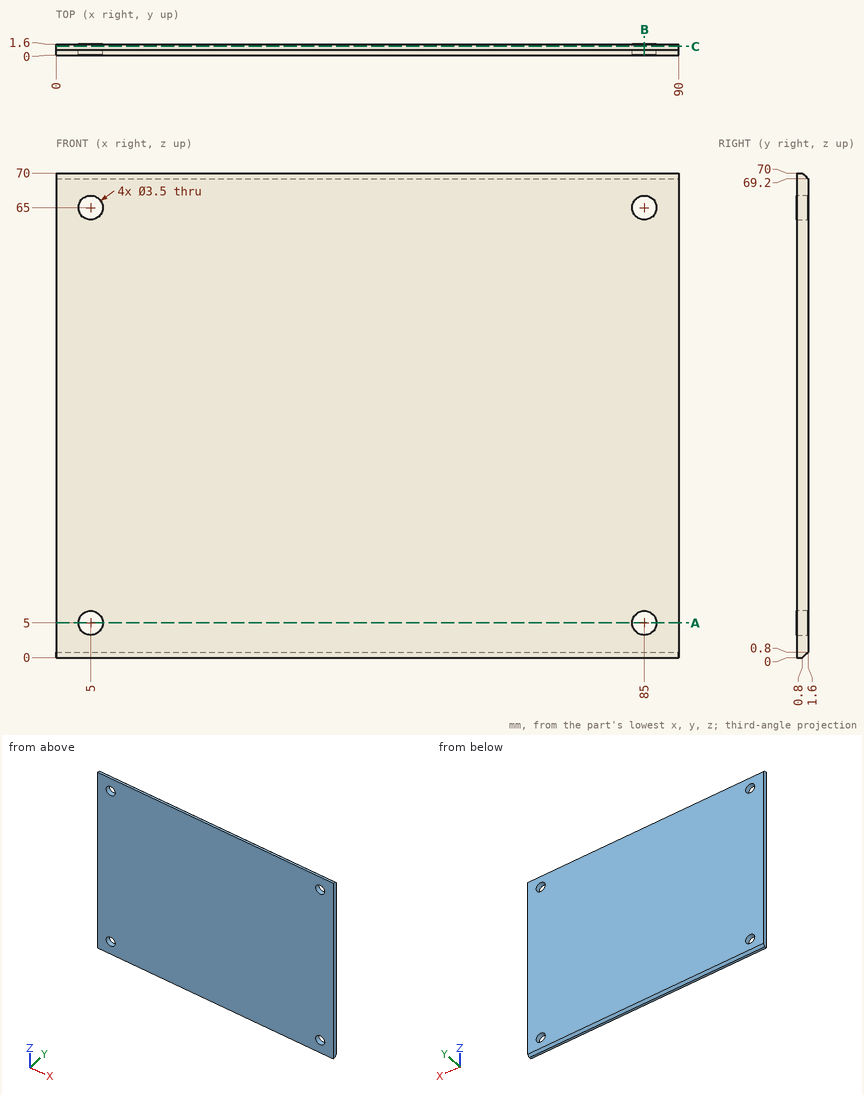
For this review, use the dimensioned drawing (mm, ordinates from the lowest corner) and the shaded views. Round coordinates to 2 decimals unless told otherwise and drop trailing zeros. Write each loop counter-clockwise with the first axis right and the second up, starting at its lowest first coordinate (ties: lowest second). Pieces come first, ordered by that corner, then holes. Notation, with made-up numbers: M -19,53 L -8,53 A19 ccw -8,79 Z; hole C 29,43 d8. An arc over 180 degrees is marked long. Use CSV: the item, a comma, the result in double quotes. Start each with the question number.
(1) We need section C-C, the plane y = 1.25. State the section outline as (x, z) points.
(2) We need section A-A, the plane z = 5. State the section outline as (x, y) points, then the cut area to 3 significant figures.
(3) We need section B-B, the plane x = 85. State the section outline as (y, z) points, then the cut area to 3 significant figures.
(4) For line 1 along X through (y, z) = (0.95, 5); line 2 along Z through (x, y) = (85, 0.6); line 3 along Z through (x, y) = (85, 1.15), list the stretches that pass through material, from the lowest coordinate up.
Findings:
1,outline,"M 0,0.45 L 90,0.45 L 90,69.55 L 0,69.55 Z; hole C 5,5 d3.5; hole C 5,65 d3.5; hole C 85,5 d3.5; hole C 85,65 d3.5"
2,outline,"M 0,0 L 3.25,0 L 3.25,1.6 L 0,1.6 Z; M 6.75,0 L 83.25,0 L 83.25,1.6 L 6.75,1.6 Z; M 86.75,0 L 90,0 L 90,1.6 L 86.75,1.6 Z"
2,area,"133 mm^2"
3,outline,"M 0,0 L 0.8,0 L 1.6,0.8 L 1.6,3.25 L 0,3.25 Z; M 0,6.75 L 1.6,6.75 L 1.6,63.25 L 0,63.25 Z; M 0,66.75 L 1.6,66.75 L 1.6,69.2 L 0.8,70 L 0,70 Z"
3,area,"100 mm^2"
4,line 1,"0 to 3.25, 6.75 to 83.25, 86.75 to 90"
4,line 2,"0 to 3.25, 6.75 to 63.25, 66.75 to 70"
4,line 3,"0.35 to 3.25, 6.75 to 63.25, 66.75 to 69.65"
